Autodesk Inventor part; units mm, degrees
ref_plane "YZ Plane" through (0, 0, 0) normal (1, 0, 0) x (0, 1, 0)
ref_plane "XZ Plane" through (0, 0, 0) normal (0, 1, 0) x (-1, 0, 0)
ref_plane "XY Plane" through (0, 0, 0) normal (0, 0, 1) x (1, 0, 0)
ref_plane "작업 평면1" through (-20.6428, -10.415, 0) normal (0, 0, 1) x (1, 0, 0)
sketch "스케치1" plane through (-20.6428, -10.415, 0) normal (0, 0, 1) x (1, 0, 0)
  arc A0 (40.7428, 14.9916) -> (40.2236, 16.6785) centre (37.7428, 14.9916) ccw
  line L0 (40.2236, 16.6785) -> (36.2381, 22.5396)
  arc A1 (36.2381, 22.5396) -> (34.5842, 23.415) centre (34.5842, 21.415) ccw
  line L1 (33.6428, 23.415) -> (34.5842, 23.415)
  arc A2 (35.1428, 21.915) -> (33.6428, 23.415) centre (33.6428, 21.915) ccw
  line L2 (35.1428, -31.085) -> (35.1428, 21.915)
  arc A3 (34.1428, -32.085) -> (35.1428, -31.085) centre (34.1428, -31.085) ccw
  line L3 (7.1428, -32.085) -> (34.1428, -32.085)
  arc A4 (6.1428, -31.085) -> (7.1428, -32.085) centre (7.1428, -31.085) ccw
  line L4 (6.1428, 21.915) -> (6.1428, -31.085)
  arc A5 (7.6428, 23.415) -> (6.1428, 21.915) centre (7.6428, 21.915) ccw
  line L5 (6.7014, 23.415) -> (7.6428, 23.415)
  arc A6 (6.7014, 23.415) -> (5.0476, 22.5396) centre (6.7014, 21.415) ccw
  line L6 (5.0476, 22.5396) -> (1.0621, 16.6785)
  arc A7 (1.0621, 16.6785) -> (0.5428, 14.9916) centre (3.5428, 14.9916) ccw
  line L7 (0.5428, 14.9916) -> (0.5428, -29.2617)
  arc A8 (0.5428, -29.2617) -> (1.0621, -30.9486) centre (3.5428, -29.2617) ccw
  line L8 (1.0621, -30.9486) -> (4.7499, -36.372)
  arc A9 (4.7499, -36.372) -> (7.2307, -37.685) centre (7.2307, -34.685) ccw
  line L9 (7.2307, -37.685) -> (34.0549, -37.685)
  arc A10 (34.0549, -37.685) -> (36.5357, -36.372) centre (34.0549, -34.685) ccw
  line L10 (36.5357, -36.372) -> (40.2236, -30.9486)
  arc A11 (40.2236, -30.9486) -> (40.7428, -29.2617) centre (37.7428, -29.2617) ccw
  line L11 (40.7428, -29.2617) -> (40.7428, 14.9916)
  circle A12 centre (3.3428, 14.415) radius 1.35
  circle A13 centre (3.3428, -7.585) radius 1.35
  circle A14 centre (9.6428, -34.885) radius 1.35
  circle A15 centre (37.9428, 14.415) radius 1.35
  circle A16 centre (37.9428, -7.585) radius 1.35
  circle A17 centre (31.6428, -34.885) radius 1.35
  circle A18 centre (3.3428, -29.585) radius 1.35
  circle A19 centre (37.9428, -29.585) radius 1.35
  line L12 (35.6928, -9.835) -> (40.1928, -9.835)
  line L13 (40.1928, -9.835) -> (40.1928, -5.335)
  line L14 (40.1928, -5.335) -> (35.6928, -5.335)
  line L15 (35.6928, -5.335) -> (35.6928, -9.835)
  line L16 (35.6928, -9.835) -> (40.1928, -5.335) construction
  line L17 (40.1928, -9.835) -> (35.6928, -5.335) construction
  line L18 (35.6928, -31.835) -> (40.1928, -31.835)
  line L19 (40.1928, -31.835) -> (40.1928, -27.335)
  line L20 (40.1928, -27.335) -> (35.6928, -27.335)
  line L21 (35.6928, -27.335) -> (35.6928, -31.835)
  line L22 (35.6928, -31.835) -> (40.1928, -27.335) construction
  line L23 (40.1928, -31.835) -> (35.6928, -27.335) construction
  point P0 (20.6428, 10.415)
  dimension "d0" = 4.5
  dimension "d1" = 4.5
  dimension "d2" = 4.5
  dimension "d3" = 4.5
extrude "돌출1" add sketch "스케치1" along normal blind 20 contours L19 L18 L10 | L10 L18 L21 L20 L19 | A16 | A19 | L15 L14 L13 L12
sketch "스케치2" plane through (19.55, -42.25, 0) normal (1, 0, 0) x (0, 0, -1)
  line L0 (0, 0) -> (0, 4.5)
  line L1 (0, 4.5) -> (-20, 4.5)
  line L2 (-20, 0) -> (-20, 4.5)
  line L3 (0, 0) -> (-20, 0)
  line L4 (0, 22) -> (0, 26.5)
  line L5 (0, 26.5) -> (-20, 26.5)
  line L6 (-20, 22) -> (-20, 26.5)
  line L7 (0, 22) -> (-20, 22)
  line L8 (-20, 0) -> (-20, 26.5)
  line L9 (-20, 26.5) -> (-15, 26.5)
  line L10 (-15, 26.5) -> (-15, 0)
  line L11 (-15, 0) -> (-20, 0)
  point P0 (0, 42.25)
  point P1 (-15, 4.5)
  point P2 (-15, 22)
  point P3 (-20, 22)
  point P4 (-20, 4.5)
  dimension "d6" = 5
extrude "돌출2" add sketch "스케치2" against normal up to surface (4.5 mm away) contours L1 L8 L7 L10
fillet "모깎기1" radius 2 2 edges at (17.3, -20.25, 15) (17.3, -37.75, 15)
fillet "모깎기2" radius 2 2 edges at (17.3, -42.25, 20) (17.3, -15.75, 20)
sketch "스케치3" plane through (-20.6428, -10.415, 0) normal (0, 0, -1) x (-1, 0, 0)
  circle A0 centre (-37.9428, -29.585) radius 1.35
  circle A1 centre (-37.9428, -7.585) radius 1.35
  circle A2 centre (-37.9428, -29.585) radius 1.05
  circle A3 centre (-37.9428, -7.585) radius 1.05
  point P0 (-20.6428, 10.415)
  dimension "d11" = 2.1
  dimension "d12" = 2.1
extrude "돌출3" cut sketch "스케치3" against normal blind 10 contours A2 | A3
sketch "스케치4" plane through (15.05, -15.75, 0) normal (0, 1, 0) x (1, 0, 0)
  line L0 (4.5, -18) -> (0, -18)
  line L1 (-30.1, -18) -> (-34.6, -18)
  line L2 (0, 0) -> (0, -18)
  line L3 (0, -18) -> (-30.1, -18)
  line L4 (2.05, -13) -> (-32.15, -13)
  line L5 (-32.15, -13) -> (-32.15, -23)
  line L6 (-32.15, -23) -> (2.05, -23)
  line L7 (2.05, -23) -> (2.05, -13)
  line L8 (2.05, -13) -> (-32.15, -23) construction
  line L9 (-32.15, -13) -> (2.05, -23) construction
  point P0 (-15.05, 0)
  point P1 (-15.05, -18)
  dimension "d15" = 34.2
  dimension "d16" = 10
extrude "돌출4" cut sketch "스케치4" against normal up to surface (26.5 mm away)
sketch "스케치5" plane through (19.55, -42.25, 0) normal (1, 0, 0) x (0, 0, -1)
  circle A0 centre (-17.3, 2.25) radius 1.35
  circle A1 centre (-17.3, 24.25) radius 1.35
  point P0 (0, 42.25)
extrude "돌출5" cut sketch "스케치5" against normal through all
sketch "스케치6" plane through (-20.6428, -10.415, 0) normal (0, 0, -1) x (-1, 0, 0)
  circle A0 centre (-37.9428, -29.585) radius 1.05
  line L0 (-35.6928, -31.835) -> (-40.1928, -31.835)
  line L1 (-35.6928, -27.335) -> (-35.6928, -31.835)
  line L2 (-40.1928, -27.335) -> (-35.6928, -27.335)
  line L3 (-40.1928, -31.835) -> (-40.1928, -27.335)
  circle A1 centre (-37.9428, -7.585) radius 1.05
  line L4 (-40.1928, -9.835) -> (-40.1928, -5.335)
  line L5 (-35.6928, -9.835) -> (-40.1928, -9.835)
  line L6 (-35.6928, -5.335) -> (-35.6928, -9.835)
  line L7 (-40.1928, -5.335) -> (-35.6928, -5.335)
  point P0 (-20.6428, 10.415)
extrude "돌출6" add sketch "스케치6" along normal blind 20
sketch "스케치7" plane through (19.55, -35.75, 15) normal (1, 0, 0) x (0, 0, -1)
  circle A0 centre (-2.3, 17.75) radius 1.35
  circle A1 centre (-2.3, -4.25) radius 1.35
  arc A2 (-3, 20) -> (-5, 18) centre (-3, 18) ccw
  line L0 (-5, -4.5) -> (-5, 18)
  arc A3 (-5, -4.5) -> (-3, -6.5) centre (-3, -4.5) ccw
  line L1 (35, -6.5) -> (-3, -6.5)
  line L2 (35, -2) -> (35, -6.5)
  line L3 (35, -2) -> (2, -2)
  arc A4 (0, 0) -> (2, -2) centre (2, 0) ccw
  line L4 (0, 0) -> (0, 13.5)
  arc A5 (2, 15.5) -> (0, 13.5) centre (2, 13.5) ccw
  line L5 (2, 15.5) -> (35, 15.5)
  line L6 (35, 20) -> (35, 15.5)
  line L7 (35, 20) -> (-3, 20)
  circle A6 centre (-2.3, 17.75) radius 1.35
  circle A7 centre (-2.3, -4.25) radius 1.35
  arc A8 (0, 0) -> (2, -2) centre (2, 0) ccw
  line L8 (2, -2) -> (2, -6.5)
  line L9 (-3, -6.5) -> (2, -6.5)
  arc A9 (-5, -4.5) -> (-3, -6.5) centre (-3, -4.5) ccw
  line L10 (-5, 18) -> (-5, -4.5)
  arc A10 (-3, 20) -> (-5, 18) centre (-3, 18) ccw
  line L11 (2, 20) -> (-3, 20)
  line L12 (2, 20) -> (2, 15.5)
  arc A11 (2, 15.5) -> (0, 13.5) centre (2, 13.5) ccw
  line L13 (0, 0) -> (0, 13.5)
  line L14 (2, -2) -> (18.5, 15.5)
  line L15 (6.1232, -2) -> (22.6232, 15.5)
  line L16 (2, 15.5) -> (18.5, -2)
  line L17 (6.1232, 15.5) -> (22.6232, -2)
  line L18 (12.3116, 4.5635) -> (12.3116, 8.9365)
  line L19 (12.3116, 8.9365) -> (0, 8.9365)
  line L20 (0, 8.9365) -> (0, 4.5635)
  line L21 (0, 4.5635) -> (12.3116, 4.5635)
  point P0 (15, 35.75)
  point P1 (14.3732, 6.75)
  point P2 (0, 8.9365)
  dimension "d23" = 3
  dimension "d24" = 3
extrude "돌출7" add sketch "스케치7" against normal up to surface (4.5 mm away) contours L19 L14 L16 | L16 L14 L21 L4 L19 | L15 L17 L14 L5 | L18 L16 L14 | L17 L15 L18 | L16 L21 L14 | L17 L3 L16 L15
sketch "스케치8" plane through (17.1, -15.75, 13) normal (-1, 0, 0) x (0, 0, 1)
  circle A0 centre (4.3, -2.25) radius 1.35
  circle A1 centre (4.3, -24.25) radius 1.35
  arc A2 (0, -22) -> (2, -20) centre (0, -20) ccw
  line L0 (0, -22) -> (0, -26.5)
  line L1 (5, -26.5) -> (0, -26.5)
  arc A3 (5, -26.5) -> (7, -24.5) centre (5, -24.5) ccw
  line L2 (7, -2) -> (7, -24.5)
  arc A4 (7, -2) -> (5, 0) centre (5, -2) ccw
  line L3 (0, 0) -> (5, 0)
  line L4 (0, 0) -> (0, -4.5)
  arc A5 (2, -6.5) -> (0, -4.5) centre (0, -6.5) ccw
  line L5 (2, -11.0635) -> (2, -6.5)
  line L6 (2, -15.4365) -> (2, -11.0635)
  line L7 (2, -20) -> (2, -15.4365)
  line L8 (0, -26.5) -> (0, -22)
  line L9 (-16.5, -22) -> (0, -22)
  line L10 (-10.3116, -15.4365) -> (-16.5, -22)
  line L11 (2, -15.4365) -> (-10.3116, -15.4365)
  line L12 (2, -11.0635) -> (2, -15.4365)
  line L13 (-10.3116, -11.0635) -> (2, -11.0635)
  line L14 (-16.5, -4.5) -> (-10.3116, -11.0635)
  line L15 (-16.5, -4.5) -> (0, -4.5)
  line L16 (0, -4.5) -> (0, 0)
  line L17 (-33, 0) -> (0, 0)
  line L18 (-33, -4.5) -> (-33, 0)
  line L19 (-33, -4.5) -> (-20.6232, -4.5)
  line L20 (-12.3732, -13.25) -> (-20.6232, -4.5)
  line L21 (-20.6232, -22) -> (-12.3732, -13.25)
  line L22 (-33, -22) -> (-20.6232, -22)
  line L23 (-33, -26.5) -> (-33, -22)
  line L24 (0, -26.5) -> (-33, -26.5)
  line L25 (-16.5, -4.5) -> (0, -4.5)
  line L26 (0, -4.5) -> (0, -22)
  point P0 (-13, 15.75)
  point P1 (0, -11.0635)
  point P2 (0, -15.4365)
extrude "돌출8" cut sketch "스케치8" along normal up to surface (2.05 mm away) contours L26 L13 L6 L11
properties part number "106_64_Connector" material "알루미늄 6061"
Input: part model. Units: mm. Frame: model coordinates. A direction names the side the tool comes from. Coordinates: 2 decimals unless noted, no trailing zeros. Write each loop counter-clockwise with the first axis right and the second up, starting at its lowest first coordinate (ties: lowest second). Pieces come first, ordered by that corner, then holes. Notation, with made-up numbers: M 74.25,-12.75 L 114.25,-12.75 A6 ccw 114.25,-7.75 Z; hole C 23,-11.5 d2. An arc over 180 degrees is marked long. Answer as a JSON object with one key per item and string values. Group by question number.
(1) Section D-D on x = 17.7. Give the number of separate pieces and of enclosed holes in the cut face, plus the area to 3 significant figures.
(2) Section B-B on y = -20.75. Output: boundary loops of the cut face in (x, z).
(3) Section A-A on z = 17.3. Output: boundary loops of the cut face in (x, y), plus the area to 3 significant figures.
(4) Section C-C on z = 1.5. Output: boundary loops of the cut face in (x, y), plus the area to 3 significant figures.
(5) Set-up query: faces 1 (the face through (17, -40, 10)), 2 (the face through (17, -26.814, 9)), 3 (the face through (16, -29, 13)). Return all of +Z, -Z, +X, -X, +Y, -Y with unobstructed straight access to the full face (end or side cutting, diameter ignored); none if empty.
(6) Ray query, line 1 along Y through (x, z) = (17.8, 12.5); line 2 along Y through (x, z) = (17.35, -14); line 3 along Y through (x, z) = (18.6, 17.3). Return the intervals inside material, ascending. Write a range as [from, to].
(7) Mould query, pull axis Z, two halves, no side actions, for faces 4 (the face through (15.05, -26, 0)), 5 (the face through (18, -17, -20)), 6 (the face through (17.33, -34.42, -0.36)), 7 (the face through (16, -18, 13)). Classes: pulls with the +Z half, pulls with the -Z half, needs draft (parallel to the pull), parting line crosses it, or undercut.
(8) Contact query for flat-ended pins moving along their axis: P1, Ø2, axis at x = 18.5, y = -33.5, coming from the -Z side; P2, Ø1, axis at x = 16.5, y = -29.5, coming from the +Z side; P3, Ø3.5, axis at y = -29.5, z = 17, coming from the -X side; P4, Ø4.5, axis at y = -18, z = 17.3, coming from the +X side. Output: stop coordinate, or through.
Result set:
{
 "1": {"separate pieces": "1", "enclosed holes": "4", "area": "441 mm2"},
 "2": {"outline": "M 15.05,-7.15 L 19.55,-7.15 L 19.55,-3.03 L 15.05,-3.03 Z; M 17.1,14.32 L 19.55,14.32 L 19.55,20 L 17.1,20 Z"},
 "3": {"outline": "M 17.1,-42.25 L 19.55,-42.25 L 19.55,-41.35 L 17.1,-41.35 Z; M 17.1,-38.65 L 19.55,-38.65 L 19.55,-19.35 L 17.1,-19.35 Z; M 17.1,-16.65 L 19.55,-16.65 L 19.55,-15.75 L 17.1,-15.75 Z", "area": "51.7 mm2"},
 "4": {"outline": "M 15.05,-42.25 L 19.55,-42.25 L 19.55,-37.75 L 15.05,-37.75 Z; M 15.05,-32.45 L 19.55,-32.45 L 19.55,-25.55 L 15.05,-25.55 Z; M 15.05,-20.25 L 19.55,-20.25 L 19.55,-15.75 L 15.05,-15.75 Z; hole C 17.3,-40 d2.1; hole C 17.3,-18 d2.1", "area": "64.6 mm2"},
 "5": {"face 1": "-Z", "face 2": "+X, -X", "face 3": "+Z, -X, +Y, -Y"},
 "6": {"line 1": "y = [-42.25, -37.75], [-31.19, -26.81], [-20.25, -15.75]", "line 2": "y = [-42.25, -41.05], [-38.95, -37.75], [-20.25, -19.05], [-16.95, -15.75]", "line 3": "y = [-42.25, -41.35], [-38.65, -19.35], [-16.65, -15.75]"},
 "7": {"face 4": "needs draft", "face 5": "pulls with the -Z half", "face 6": "undercut", "face 7": "pulls with the +Z half"},
 "8": {"P1": "stops at z = -4.56", "P2": "stops at z = 13", "P3": "stops at x = 17.1", "P4": "stops at x = 19.55"}
}
